Autodesk Fusion 360 part; units mm, degrees
sketch "Sketch1" plane through (0, 0, 0) normal (0, 0, 1) x (1, 0, 0)
  line L0 (0, 0) -> (5, 0)
  line L1 (5, 0) -> (5, -7.5)
  line L2 (5, -7.5) -> (0, -7.5)
  line L3 (0, -7.5) -> (0, 0)
  dimension "d1" = 5
  dimension "d2" = 7.5
extrude "Extrude1" add sketch "Sketch1" along normal blind 8 makes body 1
sketch "Sketch2" plane through (0, 0, 8) normal (0, 0, 1) x (-1, 0, 0)
  line L0 (0, 7.5) -> (-5, 7.5)
  line L1 (-5, 7.5) -> (-5, 0)
  line L2 (-5, 0) -> (0, 0)
  line L3 (0, 0) -> (0, 7.5)
  circle A0 centre (-2.5, 5) radius 2.5
  circle A1 centre (-2.5, 5) radius 1.75
  dimension "d5" = 3.5
extrude "Extrude2" add sketch "Sketch2" along normal blind 3 contours A0 bodies 1
sketch "Sketch3" plane through (0, 0, 0) normal (0, 0, 1) x (1, 0, 0)
  circle A0 centre (10, -5) radius 1.4
  dimension "d8" = 2.8
extrude "Extrude3" add sketch "Sketch3" along normal blind 9 separate body makes body 2
extrude "Extrude4" cut 1 faces at (2.4138, -5.3569, 8) along direction (0, 0, -1) blind 6 on bodies 1 bodies 1
sketch "Sketch4" plane through (0, 0, 0) normal (0, 0, -1) x (1, 0, 0)
  line L0 (5, 7.5) -> (0, 7.5)
  line L1 (0, 7.5) -> (0, 0)
  line L2 (0, 0) -> (5, 0)
  line L3 (5, 0) -> (5, 7.5)
  line L4 (-5, 12) -> (14, 12)
  line L5 (14, 12) -> (14, -5)
  line L6 (14, -5) -> (-5, -5)
  line L7 (-5, -5) -> (-5, 12)
extrude "Extrude5" add sketch "Sketch4" along normal blind 0.2 contours L0 L1 L2 L3 | L4 L5 L6 L7 bodies 1 2
Source: CAD feature listing. Evaluate the final solid. Frame: model axes, mm. A direction names the side the tool comes from. Coordinates: 2 decimals unless noted, no trailing zeros. Order: outer loops, then holes, each group sorted by start corner. A loop starts at its lowest first (then second) coordinate and runs counter-clockwise, first axis right, second up. Notation, with made-up numbers: (34, 89) - (57, 89) arc R10 ccw to (57, 106) - close; hole circle Ø4 at (-5, 29.5). An arc over 180 degrees is marked (long way). One line per item, written item: value.
1) Ray query, line 1 (Y direction, x = 2.5, z = 4.75); line 2 (X direction, y = -5.5, z = 5.75); line 3 (Y direction, x = 2.5, z = 9). Return the intervals inside material, ascending. Write a range as [from, to].
Computed values:
line 1: y = [-7.5, -6.75], [-3.25, 0]
line 2: x = [0, 0.82], [4.18, 5], [8.69, 11.31]
line 3: y = [-7.5, -6.75], [-3.25, -2.5]
2) Cut plane A-A on z = 4.75. Output: boundary loops of the cut face in (x, y).
Computed values:
outline: (0, -7.5) - (5, -7.5) - (5, 0) - (0, 0) - close; circle Ø2.8 at (10, -5); hole circle Ø3.5 at (2.5, -5)
3) Cut plane C-C on y = 2.25. Output: boundary loops of the cut face in (x, z), plus the area to 3 significant figures.
Computed values:
outline: (-5, -0.2) - (14, -0.2) - (14, 0) - (-5, 0) - close
area: 3.80 mm^2
4) Cut plane D-D on x = 1. Output: boundary loops of the cut face in (y, z).
Computed values:
outline: (-12, -0.2) - (5, -0.2) - (5, 0) - (0, 0) - (0, 8) - (-3, 8) - (-3, 11) - (-4.1, 11) - (-4.1, 2) - (-5.9, 2) - (-5.9, 11) - (-7, 11) - (-7, 8) - (-7.5, 8) - (-7.5, 0) - (-12, 0) - close
5) Cut plane B-B on x = 10. Output: boundary loops of the cut face in (y, z), plus the area to 3 significant figures.
Computed values:
outline: (-12, -0.2) - (5, -0.2) - (5, 0) - (-3.6, 0) - (-3.6, 9) - (-6.4, 9) - (-6.4, 0) - (-12, 0) - close
area: 28.6 mm^2
6) Contact query for flat-ended pins moving along their axis: pin 1 (1.4 mm diameter, centred on x = 10, y = -5.5, fed in from +Z); pin 2 (2 mm diameter, centred on x = 6.5, z = 7, fed in from -Y); pin 3 (3 mm diameter, centred on x = 2.5, y = -5, fed in from +Z); pin 4 (3 mm diameter, centred on y = -3.5, z = 8.5, fed in from -X). Output: stop coordinate, or through.
Computed values:
pin 1: stops at z = 9
pin 2: passes through
pin 3: stops at z = 2
pin 4: stops at x = 0
7) Reachability of faces 5 (the face through (10, -5, 9)), 6 (the face through (2, 0, 4)), 7 (the face through (3, -7.5, 4)), 8 (the face through (2, -7, 11)), 9 (the face through (2.88, -6.71, 6.44)) from +Z, -Z, +X, -X, +Y, -Y: full face, straight path, thin tool, end or side. Return the list, or none.
Computed values:
face 5: +Z, +X, +Y, -Y
face 6: +Z, +X, -X, +Y
face 7: +Z, +X, -X, -Y
face 8: +Z, +X, -X, +Y, -Y
face 9: +Z
8) Mould query, pull axis X, two halves, no side actions, for faces 1 (the face through (4.5, -7, 8)), 2 (the face through (5, -4, 4)), 3 (the face through (0, -4, 4)), 4 (the face through (0.5, -6.9, 8)). Classes: released by +X, released by -X, zero draft, split by the parting line, or undercut.
Computed values:
face 1: undercut
face 2: undercut
face 3: released by -X
face 4: zero draft
